Can you work these out from the drawing? Everything is in mm from the part's minimum corner. A direction names the side the tool comes from. Give positions to 0.01 mm unless a question says otherwise; leave off trailing zeros. Order: outer loops, then holes, each group sorted by start corner. A loop starts at its lowest first (then second) coordinate and runs counter-clockwise, first axis right, second up. Notation, with made-up numbers: (58, 87.5) -> (112, 87.5) arc R23 ccw to (112, 126.5) -> close; hole circle Ø4 at (-10.5, -29). An arc over 180 degrees is marked (long way). One line per item, written item: value.
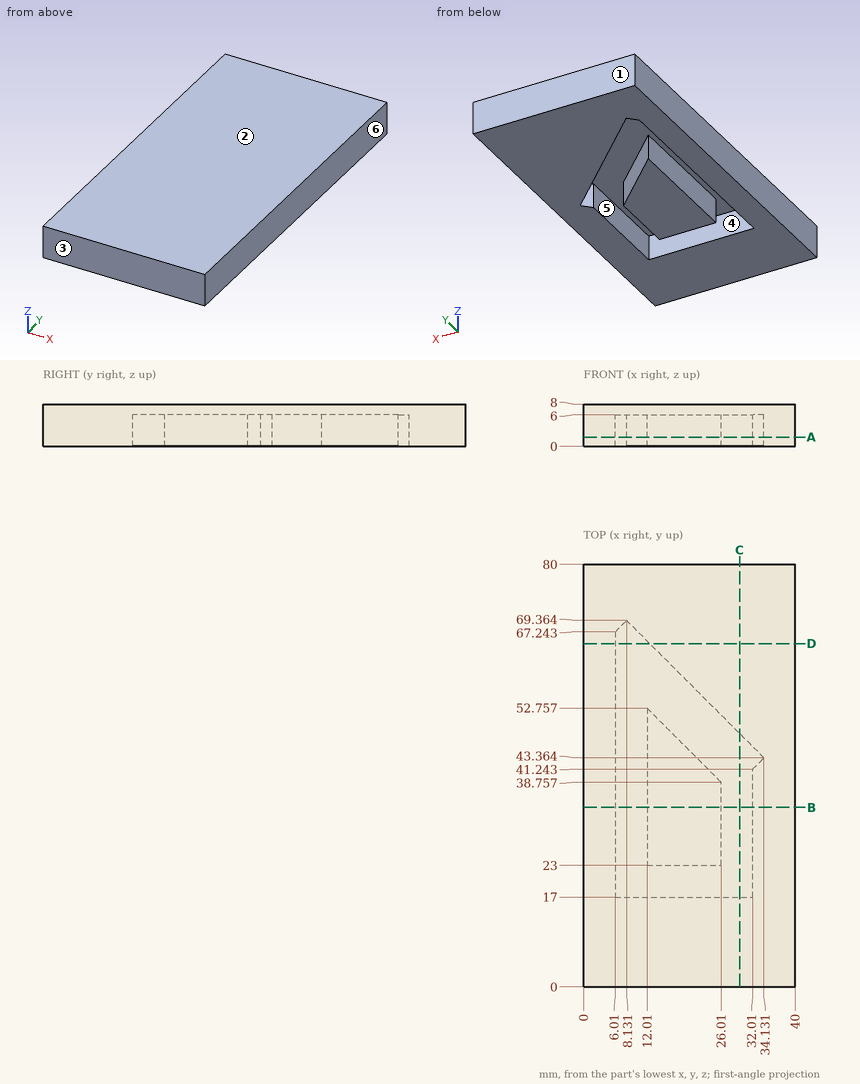
1) Suppose I cut it at A-A, the plane z = 1.75. Write out the boundary of the cut face in (x, y), then the cut area to 3 significant figures.
Answer below:
outline: (0, 0) -> (40, 0) -> (40, 80) -> (0, 80) -> close; (12.01, 23) -> (26.01, 23) -> (26.01, 38.76) -> (12.01, 52.76) -> close; hole (6.01, 17) -> (32.01, 17) -> (32.01, 41.24) -> (34.13, 43.36) -> (8.13, 69.36) -> (6.01, 67.24) -> close
area: 2,440 mm2
2) For P1, Ø1, axis at x = 30, y = 33.5, coming from the -Z side, with a flat end and sliding along its axis, tell me the tip position at first contact or that it passes through.
Answer below:
P1: stops at z = 6
3) If I drill on line 1 along X through (y, z) = (31.5, 1); line 2 along X through (y, z) = (44, 3.5) (1 decimal); line 3 along Y through (x, z) = (19, 4) (1 decimal), over which ranges is the centre line in solid material (lowest first)?
Answer below:
line 1: x = 0 to 6.01, 12.01 to 26.01, 32.01 to 40
line 2: x = 0 to 6, 12 to 20.8, 33.5 to 40
line 3: y = 0 to 17, 23 to 45.8, 58.5 to 80
4) Suppose I cut it at C-C, the plane x = 29.5. Write out the boundary of the cut face in (y, z) (1 decimal).
Answer below:
outline: (0, 0) -> (17, 0) -> (17, 6) -> (48, 6) -> (48, 0) -> (80, 0) -> (80, 8) -> (0, 8) -> close
5) We'd pull the mould along Y, two halves only. Please class the marked faces 1, 2, 3 and 4: +Y half, -Y half, draft (parallel to the pull), parting line (faces both ways), or undercut.
Answer below:
face 1: +Y half
face 2: draft
face 3: -Y half
face 4: undercut
6) For the marked faces 5 and 6, which set-ups out of +Z, -Z, +X, -X, +Y, -Y let a thin tool reach every point of the face, with its end or its side?
Answer below:
face 5: -Z
face 6: +Z, -Z, +X, +Y, -Y
7) Suppose I cut it at D-D, the plane y = 65. Write out the boundary of the cut face in (x, z) (1 decimal), then the cut area to 3 significant figures.
Answer below:
outline: (0, 0) -> (6, 0) -> (6, 6) -> (12.5, 6) -> (12.5, 0) -> (40, 0) -> (40, 8) -> (0, 8) -> close
area: 281 mm2
8) Suppose I cut it at B-B, the plane y = 34. Write out the boundary of the cut face in (x, z).
Answer below:
outline: (0, 0) -> (6.01, 0) -> (6.01, 6) -> (12.01, 6) -> (12.01, 0) -> (26.01, 0) -> (26.01, 6) -> (32.01, 6) -> (32.01, 0) -> (40, 0) -> (40, 8) -> (0, 8) -> close
